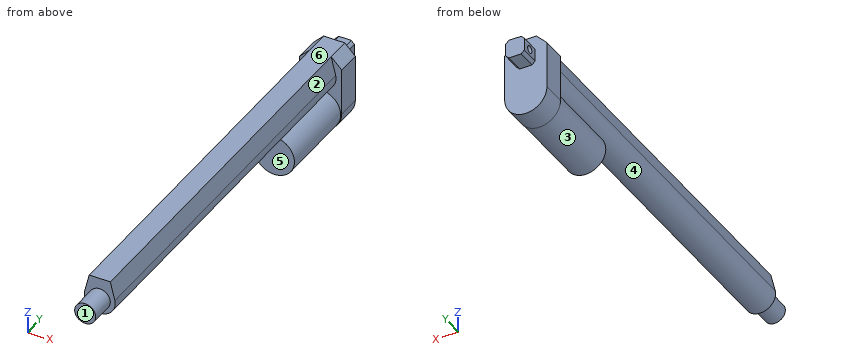
```python
from build123d import *

# Parameters (mm, degrees)
STOCK_LINEAR_ACTUATOR_CLAMPS_2026_1_DEPTH   = 369.57
STOCK_LINEAR_START                          = -24.4221
STOCK_LINEAR_ACTUATOR_CLAMPS_2026_2_R       = 9.975
STOCK_LINEAR_ACTUATOR_CLAMPS_2026_1_2_DEPTH = 24.4221
BOSS_EXTRUDE1_DEPTH                         = 22.733
SKETCH4_R                                   = 19.05
BOSS_EXTRUDE4_DEPTH                         = 77.47
CHAMFER1_SIZE                               = 10
SKETCH5_W                                   = 17.78
SKETCH5_H                                   = 17.78
BOSS_EXTRUDE5_DEPTH                         = 18.1
SKETCH6_R                                   = 3.5
CUT_EXTRUDE1_DEPTH                          = 18.1
CHAMFER2_SIZE                               = 3


# Read off the part's stored shape, not the designer's step: Stock-Linear Actuator Clamps (2026)-1
with BuildPart() as part:
    # Stock-Linear Actuator Clamps (2026)-1 ou → Stock-Linear Actuator Clamps (2026)-1 (new body)
    with BuildSketch(Plane(origin=(0, 0, 0), x_dir=(1, 0, 0), z_dir=(0, 1, 0))):
        with BuildLine():
            ThreePointArc((14.298722896, -2.925841512), (0, 14.595), (-14.298722896, -2.925841512))
            Line((-14.298722896, -2.925841512), (-10, -20.405))
            Line((-10, -20.405), (10, -20.405))
            Line((10, -20.405), (14.298722896, -2.925841512))
        make_face()
    extrude(amount=STOCK_LINEAR_ACTUATOR_CLAMPS_2026_1_DEPTH)

    # Stock-Linear Actuator Clamps _2026_- 2 → Stock-Linear Actuator Clamps _2026_-1 2 (add)
    with BuildSketch(Plane(origin=(0, 0, 0), x_dir=(1, 0, 0), z_dir=(0, 1, 0)).offset(STOCK_LINEAR_START)):
        Circle(STOCK_LINEAR_ACTUATOR_CLAMPS_2026_2_R)
    extrude(amount=STOCK_LINEAR_ACTUATOR_CLAMPS_2026_1_2_DEPTH)

    # Sketch3 → Boss-Extrude1 (add)
    with BuildSketch(Plane(origin=(0, 369.57, 0), x_dir=(1, 0, 0), z_dir=(0, 1, 0))):
        with BuildLine():
            Line((-20, -20.405), (20, -20.405))
            Line((20, -20.405), (20, 34.2075))
            ThreePointArc((20, 34.2075), (0, 54.2075), (-20, 34.2075))
            Line((-20, 34.2075), (-20, -20.405))
        make_face()
    extrude(amount=BOSS_EXTRUDE1_DEPTH)

    # Sketch4 → Boss-Extrude4 (add)
    with BuildSketch(Plane.XZ.offset(-369.57)):
        with Locations(Location((0, -35.1575, 0), (0, 0, 269.999148225))):
            Circle(SKETCH4_R)
    extrude(amount=BOSS_EXTRUDE4_DEPTH)

    # Chamfer1
    chamfer1_edges = [part.edges().sort_by_distance(p)[0] for p in [
        (-20, 380.9365, 20.405),
        (20, 380.9365, 20.405),
    ]]
    chamfer(chamfer1_edges, length=CHAMFER1_SIZE)

    # Sketch5 → Boss-Extrude5 (add)
    with BuildSketch(Plane(origin=(0, 392.303, 0), x_dir=(1, 0, 0), z_dir=(0, 1, 0))):
        with Locations((0, -1.515)):
            Rectangle(SKETCH5_W, SKETCH5_H)
    extrude(amount=BOSS_EXTRUDE5_DEPTH)

    # Sketch6 → Cut-Extrude1 (cut)
    with BuildSketch(Plane.ZY.offset(8.89)):
        with Locations((1.515, 401.353)):
            Circle(SKETCH6_R)
    extrude(amount=-CUT_EXTRUDE1_DEPTH, mode=Mode.SUBTRACT)

    # Chamfer2
    chamfer2_edges = [part.edges().sort_by_distance(p)[0] for p in [
        (-8.89, 401.353, -7.375),
        (-8.89, 401.353, 10.405),
        (8.89, 401.353, 10.405),
        (8.89, 401.353, -7.375),
    ]]
    chamfer(chamfer2_edges, length=CHAMFER2_SIZE)


solid = part.part
```
Design review of the part built by this model. Coordinates are the model's own, in mm. Face numbers are marked on the shaded views. A direction names the side the tool comes from. Give positions to 0.01 mm unless a question says otherwise; leave off trailing zeros. Write each loop counter-clockwise with the first axis right and the second up, starting at its lowest first coordinate (ties: lowest second). Pieces come first, ordered by that corner, then holes. Notation, with made-up numbers: (41, 60) -> (97, 60) arc R8 cw to (97, 72) -> close; hole circle Ø9 at (80, 65). An arc over 180 degrees is marked (long way). Answer in a Markdown table with one row per item.
(1) Mouldability with a two-part tool opening along Z and no side actions: class the marked faces 4, 5 and 6 as +Z half, -Z half, draft (parallel to the pull), parting line (faces both ways), or undercut.
Results:
| item | result |
|---|---|
| face 4 | undercut |
| face 5 | draft |
| face 6 | +Z half |
(2) Clearance check with flat-ended pins moving along their axes: pin 1 (6 mm diameter, centred on x = 5.5, z = -13, fed in from +Y); pin 2 (10 mm diameter, centred on x = 0.5, y = 202.5, fed in from -Z) (3 decimals); pin 3 (20 mm diameter, centred on x = 8.5, z = -31, fed in from -Y). State where each tip first meets the part, or that it passes through.
Results:
| item | result |
|---|---|
| pin 1 | y = 392.3 |
| pin 2 | z = -14.595 |
| pin 3 | y = 292.1 |
(3) Consider section B-B (y = 98). State the section outline as (x, z) points (3 decimals).
Results:
| item | result |
|---|---|
| outline | (-14.299, 2.926) arc R14.595 ccw (long way) to (14.299, 2.926) -> (10, 20.405) -> (-10, 20.405) -> close |
(4) Consider section A-A (z = -28). State the section outline as (x, y) points, then the cut area to 3 significant figures.
Results:
| item | result |
|---|---|
| outline | (-20, 369.57) -> (-17.65, 369.57) -> (-17.65, 292.1) -> (17.65, 292.1) -> (17.65, 369.57) -> (20, 369.57) -> (20, 392.3) -> (-20, 392.3) -> close |
| area | 3,640 mm2 |
(5) For the marked faces 1, 2 and 3, list the 3-axis set-ups (+Z, -Z, +X, -X, +Y, -Y) from which the entire face can be reached by the end or side of a thin tool; tool diameter is ignored.
Results:
| item | result |
|---|---|
| face 1 | +Z, -Z, +X, -X, -Y |
| face 2 | +Z, +X, -Y |
| face 3 | -Y |
(6) To check wall thickness, follow probe 1 along Z at (x, y) = (1, 331) (3 decimals); probe 2 along Y at (x, z) = (4, -14.5); probe 3 along Y at (x, z) = (-13.5, -45). State the ranges of each line that lie inside material, in increasing order.
Results:
| item | result |
|---|---|
| probe 1 | -54.181 to -16.134, -14.561 to 20.405 |
| probe 2 | 369.57 to 392.3 |
| probe 3 | 292.1 to 392.3 |
